```python
from build123d import *

# Parameters (mm, degrees)
SKETCH1_W           = 40
SKETCH1_H           = 100
SKETCH1_R           = 4.8
BOSS_EXTRUDE1_DEPTH = 5
SKETCH1_3_R         = 4.8
BOSS_EXTRUDE2_DEPTH = 5.2
SKETCH2_R           = 2.5
CUT_EXTRUDE1_DEPTH  = 55.809123328
SKETCH3_R           = 2.65
CUT_EXTRUDE2_DEPTH  = 5
CHAMFER1_SIZE       = 0.15
BOSS_EXTRUDE3_DEPTH = 100


with BuildPart() as part:
    # Sketch1 → Boss-Extrude1 (new body)
    # profile 1 of 3: a face of its own
    with BuildSketch(Plane.YZ):
        Rectangle(SKETCH1_W, SKETCH1_H)
        with Locations((0, -15.35)):
            Circle(SKETCH1_R, mode=Mode.SUBTRACT)
        with Locations((0, 15.35)):
            Circle(SKETCH1_R, mode=Mode.SUBTRACT)
    # profile 2 of 3: a face of its own
    with BuildSketch(Plane.YZ):
        with Locations((0, -15.35)):
            Circle(SKETCH1_R)
    # profile 3 of 3: a face of its own
    with BuildSketch(Plane.YZ):
        with Locations((0, 15.35)):
            Circle(SKETCH1_R)
    extrude(amount=BOSS_EXTRUDE1_DEPTH)

    # Sketch1<3> → Boss-Extrude2 (add)
    with BuildSketch(Plane.YZ):
        with Locations(Location((0, 15.35, 0), (0, 0, 270))):
            Circle(SKETCH1_3_R)
        with Locations(Location((0, -15.35, 0), (0, 0, 270))):
            Circle(SKETCH1_3_R)
    extrude(amount=-BOSS_EXTRUDE2_DEPTH)

    # Sketch2 → Cut-Extrude1 (cut, through all)
    with BuildSketch(Plane(origin=(-5.2, 0, 0), x_dir=(0, -1, 0), z_dir=(-1, 0, 0))):
        with Locations(Location((0, -15.35, 0), (0, 0, 90))):
            Circle(SKETCH2_R)
    extrude(amount=-CUT_EXTRUDE1_DEPTH, mode=Mode.SUBTRACT)

    # Sketch3 → Cut-Extrude2 (cut)
    with BuildSketch(Plane(origin=(5, 0, 0), x_dir=(0, 0, -1), z_dir=(1, 0, 0))):
        with Locations((15.35, 0)):
            Circle(SKETCH3_R)
    extrude(amount=-CUT_EXTRUDE2_DEPTH, mode=Mode.SUBTRACT)

    # Chamfer1
    chamfer1_edges = [part.edges().sort_by_distance(p)[0] for p in [
        (0, 0, -17.85),
    ]]
    chamfer(chamfer1_edges, length=CHAMFER1_SIZE - 0.0001)  # a hair under: the kernel refuses the full size

    # Sketch4 → Boss-Extrude3 (add)
    with BuildSketch(Plane(origin=(0, 0, -50), x_dir=(1, 0, 0), z_dir=(0, 0, -1))):
        with BuildLine():
            Line((5, -20), (0, -20))
            ThreePointArc((0, -20), (2.5, -33.538348415), (5, -20))
        make_face()
    extrude(amount=-BOSS_EXTRUDE3_DEPTH)


solid = part.part
```
Here's how the part is built. I have some questions about the finished solid (model axes, mm). A direction names the side the tool comes from. Coordinates: 2 decimals unless noted, no trailing zeros. Order: outer loops, then holes, each group sorted by start corner. A loop starts at its lowest first (then second) coordinate and runs counter-clockwise, first axis right, second up. Notation, with made-up numbers: (21.25, 85.5) -> (63.25, 85.5) arc R7 cw to (63.25, 96.5) -> close; hole circle Ø9 at (31, -8). An arc over 180 degrees is marked (long way). Return JSON: item names as keys, results as strings.
1) If we section it at D-D on y = 15: List the corners of the cut face in (x, z) for me.
Conclusion:
{"outline": "(0, -50) -> (5, -50) -> (5, 50) -> (0, 50) -> close"}
2) I'm going to push flat-ended pins straight in: P1, Ø6, axis at y = -5.5, z = -14.5, coming from the +X side; P2, Ø8, axis at x = 6, y = 1.5, coming from the +Z side; P3, Ø1, axis at x = 6.5, z = -32, coming from the +Y side; P4, Ø1, axis at y = -7, z = 15, coming from the -X side. Where does each tip first touch, or does it pass through?
Conclusion:
{"P1": "stops at x = 5", "P2": "stops at z = 50", "P3": "stops at y = 32.6", "P4": "stops at x = 0"}
3) Thinking about a two-plate mould opening in Z: for faces 1 (the flat face through (2, 12, 50)), 2 (the flat face through (-5.2, 0, 15)), 3 (the cylindrical face through (2.5, 0.1, -12.7)), which applies, +Z half, -Z half, draft (parallel to the pull), parting line (faces both ways), or undercut?
Conclusion:
{"face 1": "+Z half", "face 2": "draft", "face 3": "undercut"}
4) If I drill on probe 1 along Y at (x, z) = (2, -15.35); probe 2 along Y at (x, z) = (-2.45, -15.35); probe 3 along X at (y, z) = (10.5, -11.5), over which ranges is the centre line in solid material (lowest first)?
Conclusion:
{"probe 1": "y = -20 to -2.65, 2.65 to 33.52", "probe 2": "y = -4.8 to -2.5, 2.5 to 4.8, 21.59 to 31.49", "probe 3": "x = 0 to 5"}
5) If we section it at C-C on z = 15.35: List the corners of the cut face in (x, y) for me, plus the area to 3 significant figures.
Conclusion:
{"outline": "(-5.2, -4.8) -> (0, -4.8) -> (0, -20) -> (5, -20) -> (5, 20) arc R7 ccw (long way) to (0, 20) -> (0, 4.8) -> (-5.2, 4.8) -> close", "area": "402 mm²"}
6) On a 3-axis mill with a long thin cutter (end or side, diameter ignored), from which of +Z, -Z, +X, -X, +Y, -Y can I reach the whole of each face in a straight line? I mean faces 4 (the cylindrical face through (-2.56, 1.44, 10.77)), 5 (the flat face through (2, 12, -50)), 6 (the flat face through (5, 0, 1)). Say none if no direction works.
Conclusion:
{"face 4": "-X", "face 5": "-Z, +X, -X, +Y, -Y", "face 6": "+Z, -Z, +X, -Y"}
